from build123d import *

# Parameters (mm, degrees)
F1_DEPTH = 4
F2_W     = 2.7
F2_H     = 4
F3_DEPTH = 1.5


with BuildPart() as f1:
    # F0 (on Top) → F1 (new body)
    with BuildSketch(Plane.XY):
        Polygon((-5, -11), (5, -11), (22, -2), (22, 2), (5, 11), (-5, 11), (-22, 2), (-22, -2), align=None)
        Polygon((15.0000007647, -2.8771487377), (4.3790599258, -8.4999997701), (-4.3790599258, -8.4999997701), (-14.9999995266, -2.8771493931), (-14.9999995266, -2), (-17.5000002913, -2), (-17.5, 2), (-14.9999995266, 2), (-14.9999995266, 2.8771493931), (-4.3790599258, 8.4999997701), (4.3790599258, 8.4999997701), (15.0000007647, 2.8771487377), (15.0000007647, 2), (17.5000002913, 2), (17.5, -2), (15.0000007647, -2), align=None, mode=Mode.SUBTRACT)
    extrude(amount=F1_DEPTH)

    # F2 (on face) → F3 (cut)
    with BuildSketch(Plane(origin=(0, 0, 0), x_dir=(1, 0, 0), z_dir=(0, 0, -1))):
        with Locations((-18.85, 0)):
            Rectangle(F2_W, F2_H)
        with Locations((18.85, 0)):
            Rectangle(F2_W, F2_H)
    extrude(amount=-F3_DEPTH, mode=Mode.SUBTRACT)


solid = f1.part
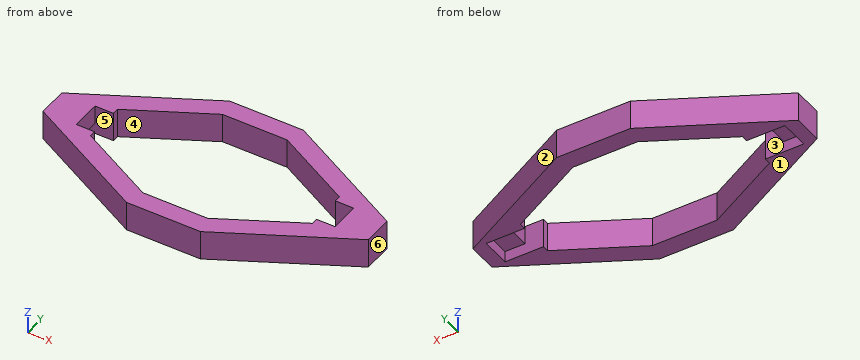
Verification items for the finished model (mm, model axes). Face numbers are marked on the shaded views. A direction names the side the tool comes from. Give positions to 0.01 mm unless a question says otherwise; leave off trailing zeros. Order: outer loops, then holes, each group sorted by start corner. A loop starts at its lowest first (then second) coordinate and runs counter-clockwise, first axis right, second up. Notation, with made-up numbers: M -24.5,89 L -12.5,89 A23 ccw -12.5,126 Z; hole C 82,-33 d5. An arc over 180 degrees is marked long. Answer as a JSON object with one key per item and string values. Group by question number.
1) Scan lines: line 1 along Y through (x, z) = (-0.5, 2.7); line 2 along X through (y, z) = (-1, 3.2); line 3 along X through (y, z) = (5, 0.85). Record each from-to range of solid material in increasing order. Write a range as [from, to].
2) Cross-section at C-C (x = 1). Enter the section's corners in (y, z), then the cut area to 3 significant figures.
3) Mould release check, pull along X, two halves, no side actions. Record for the marked faces 1, 2 and 3: released by +X, released by -X, zero draft, split by the parting line, or undercut.
4) Depth check by flat-ended pin: pin 1 Ø2 at (x, z) = (17.5, 1.5) entering from +Y; pin 2 Ø2 at (x, z) = (-17, 2) entering from -Y; pin 3 Ø1 at (x, z) = (-12, 2) entering from +Y; pin 4 Ø6 at (x, y) = (16.5, -1) entering from -Z. Enter the tip coordinate at first touch or a pass-through.
5) Access from +Z, -Z, +X, -X, +Y, -Y to the whole of each face (thin tool, end or side, straight path). Record for the marked faces 4, 5 and 6.
6) Cross-section at A-A (y = 1). Enter the section's corners in (x, z), then the cut area to 3 significant figures.
7) Cross-section at B-B (z = 2.1). Enter the section's corners in (x, y).
8) Cross-section at D-D (x = 16). Enter the section's corners in (y, z).
Result sheet:
{
 "1": {"line 1": "y = [-11, -8.5], [8.5, 11]", "line 2": "x = [-22, -17.5], [17.5, 22]", "line 3": "x = [-16.33, -10.99], [10.99, 16.33]"},
 "2": {"outline": "M -11,0 L -8.5,0 L -8.5,4 L -11,4 Z; M 8.5,0 L 11,0 L 11,4 L 8.5,4 Z", "area": "20.0 mm2"},
 "3": {"face 1": "zero draft", "face 2": "released by +X", "face 3": "undercut"},
 "4": {"pin 1": "stops at y = 4.91", "pin 2": "stops at y = -5.18", "pin 3": "stops at y = 7.56", "pin 4": "stops at z = 0"},
 "5": {"face 4": "+Z, -Z", "face 5": "-Z", "face 6": "+Z, -Z, +X, +Y, -Y"},
 "6": {"outline": "M -22,0 L -20.2,0 L -20.2,1.5 L -17.5,1.5 L -17.5,4 L -22,4 Z; M 17.5,1.5 L 20.2,1.5 L 20.2,0 L 22,0 L 22,4 L 17.5,4 Z", "area": "27.9 mm2"},
 "7": {"outline": "M -22,-2 L -5,-11 L 5,-11 L 22,-2 L 22,2 L 5,11 L -5,11 L -22,2 Z; hole M -17.5,-2 L -15,-2 L -15,-2.88 L -4.38,-8.5 L 4.38,-8.5 L 15,-2.88 L 15,-2 L 17.5,-2 L 17.5,2 L 15,2 L 15,2.88 L 4.38,8.5 L -4.38,8.5 L -15,2.88 L -15,2 L -17.5,2 Z"},
 "8": {"outline": "M -5.18,0 L -2,0 L -2,4 L -5.18,4 Z; M 2,0 L 5.18,0 L 5.18,4 L 2,4 Z"}
}
